Check sheet for the modelled part. Datum: model origin and axes. Units: mm. A direction names the side the tool comes from. Give positions to 0.01 mm unless a question says otherwise; leave off trailing zeros. Order: outer loops, then holes, each group sorted by start corner. A loop starts at its lowest first (then second) coordinate and runs counter-clockwise, first axis right, second up. Notation, with made-up numbers: (17, 12.5) -> (45, 12.5) arc R30 cw to (45, 43.5) -> close; hole circle Ø2 at (-35, 89). An arc over 180 degrees is marked (long way). Answer in a Markdown table with one row per item. Add a question column.
(1) Cross-section at C-C (x = 114). Record the cut outline in (y, z).
(2) Cross-section at B-B (y = 262). Record the cut outline in (x, z), then the cut area to 3 significant figures.
(3) Set-up check for faces 1 (the face through (25.4, 23, -336)), 2 (the face through (25.4, 226, -13)), 3 (the face through (13, 226, -25.4)), 4 (the face through (325, 13, -431.8)): record each of +Z, -Z, +X, -X, +Y, -Y from which the full face is reachable in a straight line by a thin tool's end or side.
(4) Release check for a two-part mould opening along Z. For faces 5 (the face through (232, 13, -457.2)), 6 (the face through (231, 445, -431.758)), 7 (the face through (0, 194, -433)) record: released by +Z, released by -Z, zero draft, split by the parting line, or undercut.
(5) Go/stop test with flat-tipped pins: pin 1 (20.5 mm diameter, centred on x = 258.5, z = -443, fed in from -Y); pin 2 (5 mm diameter, centred on x = 212, z = -386, fed in from +Y); pin 3 (7.5 mm diameter, centred on y = 15, z = -144, fed in from +X); pin 4 (20.5 mm diameter, centred on x = 442.5, y = 245.5, fed in from -Z). Record where each tip stops, or that it passes through.
(6) Thickness scan on L1, parallel to Y at x = 191.5, z = -353.5; L2, parallel to Z at x = 434.5, y = 304; L3, parallel to Y at x = 283, z = -20.5. Record the ranges inside material, lowest first. Write a range as [from, to].
(7) Cross-section at A-A (z = -317). Record the cut outline in (x, y), then the cut area to 3 significant figures.
Autodesk Inventor part; units mm, degrees
ref_plane "YZ Plane" through (0, 0, 0) normal (1, 0, 0) x (0, 1, 0)
ref_plane "XZ Plane" through (0, 0, 0) normal (0, 1, 0) x (-1, 0, 0)
ref_plane "XY Plane" through (0, 0, 0) normal (0, 0, 1) x (1, 0, 0)
sketch "Sketch1" plane through (0, 0, 0) normal (0, 1, 0) x (-1, 0, 0)
  line L0 (0, 0) -> (-457.2, 0)
  line L1 (-457.2, 0) -> (-457.2, -25.4)
  line L2 (-457.2, -25.4) -> (0, -25.4)
  line L3 (0, -25.4) -> (0, 0)
  line L4 (0, 0) -> (-25.4, 0)
  line L5 (-25.4, 0) -> (-25.4, -457.2)
  line L6 (-25.4, -457.2) -> (0, -457.2)
  line L7 (0, -457.2) -> (0, 0)
  line L8 (0, -457.2) -> (-457.2, -457.2)
  line L9 (-457.2, -457.2) -> (-457.2, -431.8)
  line L10 (-457.2, -431.8) -> (0, -431.8)
  line L11 (0, -431.8) -> (0, -457.2)
  line L12 (-457.2, 0) -> (-431.8, 0)
  line L13 (-431.8, 0) -> (-431.8, -457.2)
  line L14 (-431.8, -457.2) -> (-457.2, -457.2)
  line L15 (-457.2, -457.2) -> (-457.2, 0)
  dimension "d0" = 457.2
  dimension "d1" = 25.4
  dimension "d2" = 25.4
  dimension "d3" = 457.2
  dimension "d4" = 457.2
  dimension "d5" = 25.4
  dimension "d6" = 25.4
sketch "Sketch2" plane through (0, 0, 0) normal (0, 1, 0) x (-1, 0, 0)
  line L0 (0, 0) -> (-25.4, 0)
  line L1 (-25.4, 0) -> (-25.4, -25.4)
  line L2 (-25.4, -25.4) -> (0, -25.4)
  line L3 (0, -25.4) -> (0, 0)
  line L4 (0, -457.1579) -> (-25.4, -457.1579)
  line L5 (-25.4, -457.1579) -> (-25.4, -431.7579)
  line L6 (-25.4, -431.7579) -> (0, -431.7579)
  line L7 (0, -431.7579) -> (0, -457.1579)
  line L8 (-457.244, -457.1579) -> (-431.844, -457.1579)
  line L9 (-431.844, -457.1579) -> (-431.844, -431.7579)
  line L10 (-431.844, -431.7579) -> (-457.244, -431.7579)
  line L11 (-457.244, -431.7579) -> (-457.244, -457.1579)
  line L12 (-457.244, 0) -> (-431.844, 0)
  line L13 (-431.844, 0) -> (-431.844, -25.4)
  line L14 (-431.844, -25.4) -> (-457.244, -25.4)
  line L15 (-457.244, -25.4) -> (-457.244, 0)
  dimension "d7" = 25.4
  dimension "d8" = 25.4
  dimension "d9" = 25.4
  dimension "d10" = 25.4
  dimension "d11" = 25.4
  dimension "d12" = 25.4
  dimension "d13" = 25.4
  dimension "d14" = 25.4
sketch "Sketch3" plane through (0, 0, 0) normal (0, 0, 1) x (1, 0, 0)
  point P0 (0, 0)
sketch "Sketch4" plane through (0, 0, 0) normal (0, 0, 1) x (1, 0, 0)
  point P0 (0, 0)
extrude "Extrusion1" add sketch "Sketch1" along normal blind 25.4 contours L3 L2 L5 L0 | L5 L2 L13 L0 | L7 L10 L5 L2 | L13 L2 L1 L0 | L7 L6 L5 L10 | L13 L10 L15 L2 | L5 L8 L13 L10 | L13 L8 L9 L10
extrude "Extrusion2" add sketch "Sketch2" along normal blind 457.2
sketch "Sketch5" plane through (0, 457.2, 0) normal (0, 1, 0) x (1, 0, 0)
  line L0 (0, 0) -> (25.4, 0)
  line L1 (25.4, 0) -> (25.4, 25.4)
  line L2 (25.4, 25.4) -> (0, 25.4)
  line L3 (0, 25.4) -> (0, 0)
  line L4 (0, 457.1579) -> (25.4, 457.1579)
  line L5 (25.4, 457.1579) -> (25.4, -0.0421)
  line L6 (25.4, -0.0421) -> (0, -0.0421)
  line L7 (0, -0.0421) -> (0, 457.1579)
  line L8 (457.244, 25.4) -> (431.844, 25.4)
  line L9 (0, 0) -> (457.2, 0)
  line L10 (457.2, 0) -> (457.2, 25.4)
  line L11 (457.2, 25.4) -> (0, 25.4)
  line L12 (0, 25.4) -> (0, 0)
  line L13 (431.844, 431.7579) -> (457.244, 431.7579)
  line L14 (0, 457.1579) -> (457.2, 457.1579)
  line L15 (457.2, 457.1579) -> (457.2, 431.7579)
  line L16 (457.2, 431.7579) -> (0, 431.7579)
  line L17 (0, 431.7579) -> (0, 457.1579)
  line L18 (457.244, 0) -> (431.844, 0)
  line L19 (431.844, 0) -> (431.844, 457.2)
  line L20 (431.844, 457.2) -> (457.244, 457.2)
  line L21 (457.244, 457.2) -> (457.244, 0)
  dimension "d19" = 25.4
  dimension "d20" = 457.2
  dimension "d21" = 457.2
  dimension "d22" = 457.2
  dimension "d23" = 25.4
  dimension "d24" = 457.2
extrude "Extrusion3" add sketch "Sketch5" against normal blind 25.4 contours L3 L2 L1 L0 | L0 L5 L6 L7 | L1 L11 L19 L9 | L7 L16 L5 L2 | L19 L8 L10 L9 | L7 L4 L5 L16 | L5 L14 L19 L16 | L19 L13 L21 L8 | L10 L8 L21 L18 | L19 L14 L15 L13 | L19 L20 L21 L13 L15 L14
sketch "Sketch6" plane through (457.244, 0, 0) normal (1, 0, 0) x (0, 0, -1)
  point P0 (0, 0)
sketch "Sketch7" plane through (0, 25.4, 0) normal (0, 1, 0) x (1, 0, 0)
  line L0 (457.2, 457.2) -> (0, 457.2)
  line L1 (190.1658, 457.2) -> (215.5658, 457.2)
  line L2 (215.5658, 457.2) -> (215.5658, 0)
  line L3 (215.5658, 0) -> (190.1658, 0)
  line L4 (190.1658, 0) -> (190.1658, 457.2)
  point P0 (0, 0)
  dimension "d27" = 25.4
  dimension "d28" = 457.2
extrude "Extrusion4" add sketch "Sketch7" against normal blind 25.4
sketch "Sketch8" plane through (0, 25.4, 0) normal (0, 1, 0) x (1, 0, 0)
  line L0 (190.1658, 431.8) -> (215.5658, 431.8)
  line L1 (215.5658, 431.8) -> (215.5658, 25.4)
  line L2 (190.1658, 25.4) -> (215.5658, 25.4)
  line L3 (190.1658, 25.4) -> (190.1658, 431.8)
  point P0 (0, 0)
properties part number "Basic Frame" material "Aluminum 6061, Welded"
Answer below:
| question | item | result |
|---|---|---|
| 1 | outline | (0, -457.2) -> (25.4, -457.2) -> (25.4, -431.8) -> (0, -431.8) -> close; (0, -25.4) -> (25.4, -25.4) -> (25.4, 0) -> (0, 0) -> close; (431.8, -457.16) -> (457.2, -457.16) -> (457.2, -431.76) -> (431.8, -431.76) -> close; (431.8, -25.4) -> (457.2, -25.4) -> (457.2, 0) -> (431.8, 0) -> close |
| 2 | outline | (0, -457.16) -> (25.4, -457.16) -> (25.4, -431.76) -> (0, -431.76) -> close; (0, -25.4) -> (25.4, -25.4) -> (25.4, 0) -> (0, 0) -> close; (431.84, -457.16) -> (457.24, -457.16) -> (457.24, -431.76) -> (431.84, -431.76) -> close; (431.84, -25.4) -> (457.24, -25.4) -> (457.24, 0) -> (431.84, 0) -> close |
| 2 | area | 2,580 mm² |
| 3 | face 1 | none |
| 3 | face 2 | +Z, -Z |
| 3 | face 3 | +X, -X |
| 3 | face 4 | +Y, -Y |
| 4 | face 5 | released by -Z |
| 4 | face 6 | undercut |
| 4 | face 7 | zero draft |
| 5 | pin 1 | stops at y = 0 |
| 5 | pin 2 | stops at y = 25.4 |
| 5 | pin 3 | stops at x = 457.2 |
| 5 | pin 4 | stops at z = -457.16 |
| 6 | L1 | y = [0, 25.4] |
| 6 | L2 | z = [-457.16, -431.76], [-25.4, 0] |
| 6 | L3 | y = [0, 25.4], [431.8, 457.2] |
| 7 | outline | (0, 0) -> (25.4, 0) -> (25.4, 25.4) -> (0, 25.4) -> close; (0, 431.8) -> (25.4, 431.8) -> (25.4, 457.2) -> (0, 457.2) -> close; (190.17, 0) -> (215.57, 0) -> (215.57, 25.4) -> (190.17, 25.4) -> close; (431.8, 0) -> (457.2, 0) -> (457.2, 25.4) -> (431.8, 25.4) -> close; (431.84, 431.8) -> (457.24, 431.8) -> (457.24, 457.2) -> (431.84, 457.2) -> close |
| 7 | area | 3,230 mm² |
